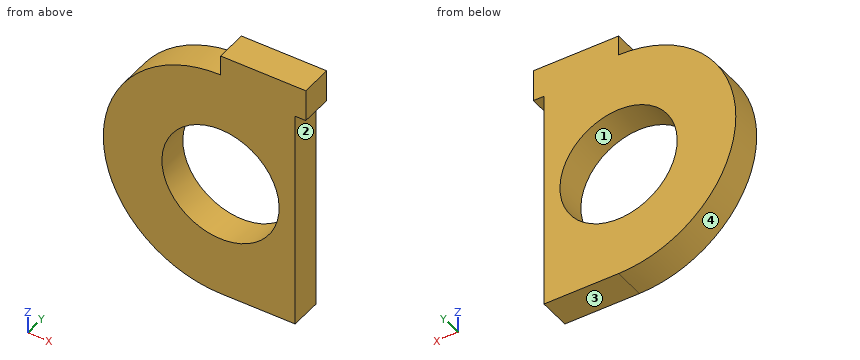
```python
from build123d import *

# Parameters (mm, degrees)
SKETCH1_R           = 11
BOSS_EXTRUDE1_DEPTH = 6


with BuildPart() as part:
    # Sketch1 → Boss-Extrude1 (new body)
    with BuildSketch(Plane(origin=(0, 0, 0), x_dir=(1, 0, 0), z_dir=(0, 1, 0))):
        with BuildLine():
            Line((0, 0), (0, 41.8))
            Line((0, 41.8), (-14, 41.8))
            ThreePointArc((-14, 41.8), (-36, 19.8), (-14, -2.2))
            Line((-14, -2.2), (-14, -6))
            Line((-14, -6), (2, -6))
            Line((2, -6), (2, 0))
            Line((2, 0), (0, 0))
        make_face()
        with Locations(Location((-14, 19.8, 0), (0, 0, 270))):
            Circle(SKETCH1_R, mode=Mode.SUBTRACT)
    extrude(amount=BOSS_EXTRUDE1_DEPTH)


solid = part.part
```
For this review, take the finished solid that the model builds, in its own axes (mm). Face numbers are marked on the shaded views. Coordinates: 2 decimals unless noted, no trailing zeros. Order: outer loops, then holes, each group sorted by start corner. A loop starts at its lowest first (then second) coordinate and runs counter-clockwise, first axis right, second up. Notation, with made-up numbers: (61.5, 61.25) - (87.5, 61.25) arc R13 ccw to (87.5, 80.25) - close; hole circle Ø3 at (-29, 37.25). An arc over 180 degrees is marked (long way). Answer as a JSON object with one key per item and string values. Group by question number.
1. We need section D-D on z = 3.5. State the section outline as (x, y) points, then the cut area to 3 significant figures.
2. We need section A-A on z = -19.8. State the section outline as (x, y) points, then the cut area to 3 significant figures.
3. We need section C-C on y = 4.9. State the section outline as (x, z) points.
4. Clearance check with flat-ended pins moving along their axes: P1, Ø8, axis at x = -30, z = -27.5, coming from the -Y side; P2, Ø2, axis at x = -28, y = 5, coming from the -Z side; P3, Ø0.6, axis at x = 1, y = 3.5, coming from the -Z side. State where each tip first meets the part, or that it passes through.
5. For probe 1 along X at (y, z) = (2.65, -19.8); probe 2 along X at (y, z) = (3.6, -13); probe 3 along Z at (x, y) = (-21, 3.2), list the stretches that pass through material, from the lowest coordinate up.
6. The part is to be moulded in two halves that separate along Z. For the marked faces 1, 2, 3 and 4, say which applies: pulls with the +Z half, pulls with the -Z half, needs draft (parallel to the pull), parting line crosses it, or undercut.
7. We need section B-B on x = -15.5. State the section outline as (y, z) points, then the cut area to 3 significant figures.
Final values:
{
 "1": {"outline": "(-14, 0) - (2, 0) - (2, 6) - (-14, 6) - close", "area": "96.0 mm²"},
 "2": {"outline": "(-36, 0) - (-25, 0) - (-25, 6) - (-36, 6) - close; (-3, 0) - (0, 0) - (0, 6) - (-3, 6) - close", "area": "84.0 mm²"},
 "3": {"outline": "(-14, -41.8) - (0, -41.8) - (0, 0) - (2, 0) - (2, 6) - (-14, 6) - (-14, 2.2) arc R22 ccw to start; hole circle Ø22 at (-14, -19.8)"},
 "4": {"P1": "y = 0", "P2": "z = -37.55", "P3": "z = 0"},
 "5": {"probe 1": "-36 to -25, -3 to 0", "probe 2": "-34.92 to -22.65, -5.35 to 0", "probe 3": "-40.66 to -28.29, -11.31 to 1.06"},
 "6": {"face 1": "undercut", "face 2": "needs draft", "face 3": "pulls with the -Z half", "face 4": "parting line crosses it"},
 "7": {"outline": "(0, -41.75) - (6, -41.75) - (6, -30.7) - (0, -30.7) - close; (0, -8.9) - (6, -8.9) - (6, 2.15) - (0, 2.15) - close", "area": "133 mm²"}
}
